from build123d import *

# Parameters (mm, degrees)
POCKET_DEPTH       = 145.459123
POCKET_DEPTH_BACK  = 177.459123
POLARPATTERN_COUNT = 5


with BuildPart() as part:
    # Sketch009 → Revolution (revolve)
    with BuildSketch(Plane.YZ):
        with BuildLine():
            Line((-32, 25), (-31.006334, 25))
            Line((-31.006334, 24), (-31.006334, 25))
            Line((-15.98482, 24), (-31.006334, 24))
            Line((-15.98482, 25), (-15.98482, 24))
            Line((-15.98482, 25), (-14.98482, 25))
            Line((-14.98482, 25), (-14.98482, 21.997654))
            ThreePointArc((-15.998639, 21.00955), (-15.282862, 21.289299), (-14.98482, 21.997654))
            Line((-15.998639, 21.00955), (-25.00382, 21.00955))
            ThreePointArc((-25.00382, 21.00955), (-25.68626, 20.700427), (-25.977919, 20.010342))
            Line((-25.977919, 2.4), (-25.977919, 20.010342))
            Line((-28.777919, 2.4), (-25.977919, 2.4))
            Line((-28.777919, 0.8), (-28.777919, 2.4))
            Line((-30.377919, 0.8), (-28.777919, 0.8))
            Line((-30.377919, 1.7), (-30.377919, 0.8))
            Line((-32, 1.7), (-30.377919, 1.7))
            Line((-32, 25), (-32, 1.7))
        make_face()
    revolve(axis=Axis((0, 0, 0), (0, 1, 0)))

    # Sketch010 → Pocket (cut, two sides)
    with BuildSketch(Plane(origin=(-5.2, 0, 0), x_dir=(1, 0, 0), z_dir=(0, -1, 0))) as pocket_sk:
        with BuildLine():
            add(Edge.make_bspline(
                [(11.995053, 15.000581), (5.131915, -6.987182), (-1.338915, 15.000254)],
                knots=[-6.684799, -6.684799, -6.684799, 6.648635, 6.648635, 6.648635], degree=2))
            ThreePointArc((-1.338915, 15.000254), (5.328035, 16.380749), (11.995053, 15.000581))
        make_face()
    pocket = extrude(amount=-POCKET_DEPTH, mode=Mode.SUBTRACT) + extrude(pocket_sk.sketch, amount=POCKET_DEPTH_BACK, mode=Mode.SUBTRACT)

    # PolarPattern: Pocket ×5 about axis
    polarpattern_axis = Axis((0, 0, 0), (0, 1, 0))
    for i in range(1, POLARPATTERN_COUNT):
        add(pocket.rotate(polarpattern_axis, i * 360 / POLARPATTERN_COUNT), mode=Mode.SUBTRACT)


with BuildPart() as part_1:
    # Body007 placement: moved
    add(part.part.moved(Location((5.2, 0, 0))))


solid = part_1.part
Read the model definition and answer for the solid it produces. Units are mm, in the model's axes. A direction names the side the tool comes from. Coordinates: 2 decimals unless noted, no trailing zeros. Loops run counter-clockwise (first coordinate to the right, second up) from the corner with the lowest first, then second, coordinate; pieces in that order, holes last.
Q1. Each of these flat-tipped pins is pushed along its axis until it touches: pin 1 Ø2 at (x, y) = (-13, -28) entering from -Z; pin 2 Ø6 at (x, y) = (3.5, -20) entering from -Z; pin 3 Ø4 at (x, y) = (-7.5, -25) entering from -Z. Where does it stop, or does it pass through?
Q2. The mould has two halves that part along Y. Classify faces 5 (the face through (1, -25.978, 0)), 6 (the face through (29, -23.6, -3.1)), 7 (the face through (-17, -15.5, 11.5)): +Y half, -Y half, draft (parallel to the pull), parting line (faces both ways), or undercut.
Q3. Consider probe 1 along X at (y, z) = (-29.15, 0); probe 2 along Y at (x, z) = (25.5, -14); probe 3 along X at (y, z) = (-21.75, 0). Determine where each line is inside the solid, lowest interval first.
Q4. Which of the six approach directions +Z, -Z, +X, -X, +Y, -Y give full straight-line access (tool end or side, diameter ignored) to faces 1 (the face through (14.6, -31.006, 22.3)), 2 (the face through (6, -28.778, 1)), 3 (the face through (5.23, -28.95, 16.38)), 4 (the face through (5, -30.378, 1))?
Q5. The part is cut by section B-B on y = -18. Write down the section's boundary in (x, z).
Q6. The part is cut by section A-A on x = 5.2. Give the number of separate pieces and of enclosed holes in the cut face, and give its area (3 significant figures).
Results below:
1. pin 1: stops at z = -16.74
1. pin 2: stops at z = -24
1. pin 3: stops at z = -21.48
2. face 5: +Y half
2. face 6: undercut
2. face 7: draft
3. probe 1: x = -18.8 to -11.16, 0.38 to 4.4, 6 to 9.95, 21.64 to 29.2
3. probe 2: y = -32 to -31.01, -15.98 to -14.98
3. probe 3: x = -18.8 to -15.81, 26.21 to 29.2
4. face 1: none
4. face 2: +Y
4. face 3: +Y, -Y
4. face 4: -Y
5. outline: circle Ø48 at (5.2, 0); hole circle Ø42.02 at (5.2, 0)
6. separate pieces: 3
6. enclosed holes: 0
6. area: 263 mm2
